from build123d import *

# Parameters (mm, degrees)
SKETCH1_W           = 80
SKETCH1_H           = 40
SKETCH1_R           = 1.15
SKETCH1_W_2         = 11.5
SKETCH1_H_2         = 11.5
SKETCH1_W_3         = 16
SKETCH1_H_3         = 14
BOSS_EXTRUDE1_DEPTH = 3
FILLET1_R           = 5


with BuildPart() as part:
    # Sketch1 → Boss-Extrude1 (new body)
    with BuildSketch(Plane.XY):
        Rectangle(SKETCH1_W, SKETCH1_H)
        with Locations((-11.5, 5)):
            Circle(SKETCH1_R, mode=Mode.SUBTRACT)
        with Locations((-11.5, -7.5)):
            Circle(SKETCH1_R, mode=Mode.SUBTRACT)
        with Locations((-33, 5)):
            Circle(SKETCH1_R, mode=Mode.SUBTRACT)
        with Locations((-33, -7.5)):
            Circle(SKETCH1_R, mode=Mode.SUBTRACT)
        with Locations((10.15, 7.45)):
            Circle(SKETCH1_R, mode=Mode.SUBTRACT)
        with Locations((10.15, -6.05)):
            Circle(SKETCH1_R, mode=Mode.SUBTRACT)
        with Locations((32.15, 7.45)):
            Circle(SKETCH1_R, mode=Mode.SUBTRACT)
        with Locations((32.15, -6.05)):
            Circle(SKETCH1_R, mode=Mode.SUBTRACT)
        with Locations((-22.25, 0.45)):
            Rectangle(SKETCH1_W_2, SKETCH1_H_2, mode=Mode.SUBTRACT)
        with Locations((21.15, 0.45)):
            Rectangle(SKETCH1_W_3, SKETCH1_H_3, mode=Mode.SUBTRACT)
    extrude(amount=BOSS_EXTRUDE1_DEPTH)

    # Fillet1
    fillet1_edges = [part.edges().sort_by_distance(p)[0] for p in [
        (40, -20, 1.5),
        (-40, -20, 1.5),
        (-40, 20, 1.5),
        (40, 20, 1.5),
    ]]
    fillet(fillet1_edges, radius=FILLET1_R)


solid = part.part
Geometry: final body of the model. Coordinates: model frame, mm. A direction names the side the tool comes from. Coordinates: 2 decimals unless noted, no trailing zeros. Order: outer loops, then holes, each group sorted by start corner. A loop starts at its lowest first (then second) coordinate and runs counter-clockwise, first axis right, second up. Notation, with made-up numbers: M -22,78 L 0,78 A17 cw 0,84 Z; hole C 36.5,79.5 d3. An arc over 180 degrees is marked long. One line per question, with ' | ' between items. Start each with the question number.
Item 1: Cut plane A-A, the plane y = -4. Return the cut outline in (x, z).
Item 2: Cut plane B-B, the plane x = 32.15. Return the cut outline in (y, z), then the cut area to 3 significant figures.
Item 3: Ray query, probe 1 along Y at (x, z) = (-11.5, 1.8); probe 2 along X at (y, z) = (1, 1.15); probe 3 along Y at (x, z) = (32.15, 1.7). Return the intervals inside material, ascending. Write a range as [from, to].
Item 4: Cut plane C-C, the plane z = 2.15. Count the separate pieces of the cut face and the enclosed holes in it, then the cut area to 3 significant figures.
Item 5: Draft query along Y for faces 3 (the cylindrical face through (38, 19, 2)), 4 (the flat face through (-16.5, 0, 1)), 5 (the flat face through (-40, 0, 1)). Return one class per face: released by +Y, released by -Y, zero draft, split by the parting line, or undercut.
Item 6: Set-up query: faces 1 (the flat face through (40, 0, 1)), 2 (the flat face through (21, -6.55, 1)). Return all of +Z, -Z, +X, -X, +Y, -Y with unobstructed straight access to the full face (end or side cutting, diameter ignored); none if empty.
A:
1) outline: M -40,0 L -28,0 L -28,3 L -40,3 Z; M -16.5,0 L 13.15,0 L 13.15,3 L -16.5,3 Z; M 29.15,0 L 40,0 L 40,3 L 29.15,3 Z
2) outline: M -20,0 L -7.2,0 L -7.2,3 L -20,3 Z; M -4.9,0 L 6.3,0 L 6.3,3 L -4.9,3 Z; M 8.6,0 L 20,0 L 20,3 L 8.6,3 Z | area: 106 mm2
3) probe 1: y = [-20, -8.65], [-6.35, 3.85], [6.15, 20] | probe 2: x = [-40, -28], [-16.5, 13.15], [29.15, 40] | probe 3: y = [-20, -7.2], [-4.9, 6.3], [8.6, 20]
4) separate pieces: 1 | enclosed holes: 10 | area: 2,790 mm2
5) face 3: released by +Y | face 4: undercut | face 5: zero draft
6) face 1: +Z, -Z, +X, +Y, -Y | face 2: +Z, -Z
